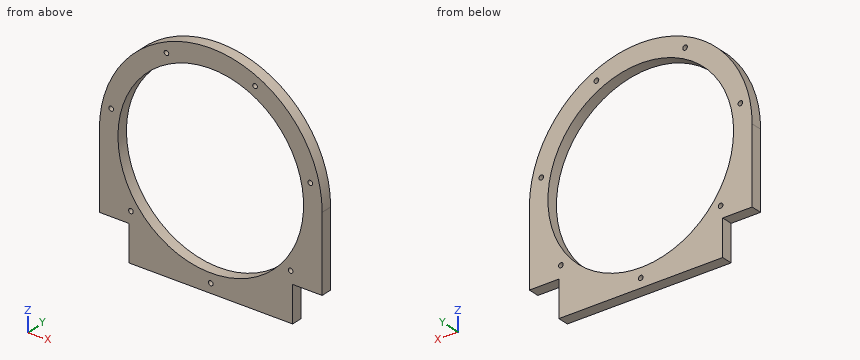
from build123d import *

# Parameters (mm, degrees)
SKETCH1_R           = 1
BOSS_EXTRUDE1_DEPTH = 4.7625


with BuildPart() as part:
    # Sketch1 → Boss-Extrude1 (new body)
    # profile 1 of 6: a face of its own
    with BuildSketch(Plane(origin=(0, 0, 0), x_dir=(1, 0, 0), z_dir=(0, 1, 0))):
        with BuildLine():
            ThreePointArc((-35.3, 32.525528435), (-19.271411924, 43.961490903), (0, 48))
            Line((0, 48), (-35.3, 48))
            Line((-35.3, 48), (-35.3, 32.525528435))
        make_face()
    # profile 2 of 6: a face of its own
    with BuildSketch(Plane(origin=(0, 0, 0), x_dir=(1, 0, 0), z_dir=(0, 1, 0))):
        with BuildLine():
            ThreePointArc((-48, 0), (-44.712414383, 17.458522274), (-35.3, 32.525528435))
            Line((-35.3, 32.525528435), (-48, 32.525528435))
            Line((-48, 32.525528435), (-48, 0))
        make_face()
    # profile 3 of 6: a face of its own
    with BuildSketch(Plane(origin=(0, 0, 0), x_dir=(1, 0, 0), z_dir=(0, 1, 0))):
        with BuildLine():
            ThreePointArc((35.3, 32.525528435), (19.271411924, 43.961490903), (0, 48))
            ThreePointArc((0, 48), (-19.271411924, 43.961490903), (-35.3, 32.525528435))
            ThreePointArc((-35.3, 32.525528435), (-44.712414383, 17.458522274), (-48, 0))
            Line((-48, 0), (-40, 0))
            ThreePointArc((-40, 0), (0, 40), (40, 0))
            Line((40, 0), (48, 0))
            ThreePointArc((48, 0), (44.712414383, 17.458522274), (35.3, 32.525528435))
        make_face()
        with Locations(Location((-34.400585229, 27.433551282, 0), (0, 0, 90))):
            Circle(SKETCH1_R, mode=Mode.SUBTRACT)
        with Locations(Location((0, 44, 0), (0, 0, 90))):
            Circle(SKETCH1_R, mode=Mode.SUBTRACT)
        with Locations(Location((34.400585229, 27.433551282, 0), (0, 0, 90))):
            Circle(SKETCH1_R, mode=Mode.SUBTRACT)
    # profile 4 of 6: a face of its own
    with BuildSketch(Plane(origin=(0, 0, 0), x_dir=(1, 0, 0), z_dir=(0, 1, 0))):
        with BuildLine():
            ThreePointArc((-48, 0), (0, -48), (48, 0))
            Line((48, 0), (40, 0))
            ThreePointArc((40, 0), (0, -40), (-40, 0))
            Line((-40, 0), (-48, 0))
        make_face()
        with Locations(Location((-19.090884521, -39.642630188, 0), (0, 0, 90))):
            Circle(SKETCH1_R, mode=Mode.SUBTRACT)
        with Locations(Location((-42.896828136, -9.790921094, 0), (0, 0, 90))):
            Circle(SKETCH1_R, mode=Mode.SUBTRACT)
        with Locations(Location((19.090884521, -39.642630188, 0), (0, 0, 90))):
            Circle(SKETCH1_R, mode=Mode.SUBTRACT)
        with Locations(Location((42.896828136, -9.790921094, 0), (0, 0, 90))):
            Circle(SKETCH1_R, mode=Mode.SUBTRACT)
    # profile 5 of 6: a face of its own
    with BuildSketch(Plane(origin=(0, 0, 0), x_dir=(1, 0, 0), z_dir=(0, 1, 0))):
        with BuildLine():
            Line((48, 32.525528435), (35.3, 32.525528435))
            ThreePointArc((35.3, 32.525528435), (44.712414383, 17.458522274), (48, 0))
            Line((48, 0), (48, 32.525528435))
        make_face()
    # profile 6 of 6: a face of its own
    with BuildSketch(Plane(origin=(0, 0, 0), x_dir=(1, 0, 0), z_dir=(0, 1, 0))):
        with BuildLine():
            Line((35.3, 48), (0, 48))
            ThreePointArc((0, 48), (19.271411924, 43.961490903), (35.3, 32.525528435))
            Line((35.3, 32.525528435), (35.3, 48))
        make_face()
    extrude(amount=BOSS_EXTRUDE1_DEPTH)


solid = part.part
Geometry: final body of the model. Coordinates: model frame, mm. Give positions to 0.01 mm unless a question says otherwise; leave off trailing zeros. Write each loop counter-clockwise with the first axis right and the second up, starting at its lowest first coordinate (ties: lowest second). Pieces come first, ordered by that corner, then holes. Notation, with made-up numbers: (-17.5, 69.5) - (28.5, 69.5) arc R15 cw to (28.5, 78.5) - close; hole circle Ø4 at (3.25, -2.5). An arc over 180 degrees is marked (long way). Return JSON: item names as keys, results as strings. Group by question number.
1) Section C-C on y = 3.55. State how many separate pieces and enclosed holes the cut face has, plus the area to 3 significant figures.
2) First-contact query: P1, Ø2.5, axis at x = -43.5, y = 3, coming from the -Z side; P2, Ø2, axis at y = 2.5, z = -37.5, coming from the -X side. Flat tips, straight axial feed; report the tip coordinate or a pass-through.
3) Section A-A on x = 16.5. Return the cut outline in (y, z), plus the area to 3 significant figures.
4) Section B-B on z = 29.5. Return the cut outline in (x, y).
5) Line query: line 1 (Z direction, x = -18.5, y = 1.65); line 2 (Z direction, x = -33.5, y = 3.8); line 3 (X direction, y = 1.05, z = -27). Output: solid intervals per line, ascending.
Filled in:
{
 "1": {"separate pieces": "1", "enclosed holes": "8", "area": "2,790 mm^2"},
 "2": {"P1": "stops at z = -32.53", "P2": "stops at x = -35.3"},
 "3": {"outline": "(0, -48) - (4.76, -48) - (4.76, -36.44) - (0, -36.44) - close; (0, 36.44) - (4.76, 36.44) - (4.76, 45.07) - (0, 45.07) - close", "area": "96.2 mm^2"},
 "4": {"outline": "(-37.86, 0) - (-27.01, 0) - (-27.01, 4.76) - (-37.86, 4.76) - close; (27.01, 0) - (37.86, 0) - (37.86, 4.76) - (27.01, 4.76) - close"},
 "5": {"line 1": "z = -48 to -35.46, 35.46 to 38.84, 40.45 to 44.29", "line 2": "z = -48 to -27.87, -27 to -21.86, 21.86 to 34.38", "line 3": "x = -48 to -35.3, -33.5 to -29.51, 29.51 to 33.5, 35.3 to 48"}
}
